Geometry check sheet. Reference: the model listing, model coordinates, mm. A direction names the side the tool comes from. Give positions to 0.01 mm unless a question says otherwise; leave off trailing zeros. Loops run counter-clockwise (first coordinate to the right, second up) from the corner with the lowest first, then second, coordinate; pieces in that order, holes last.
```python
from build123d import *

# Parameters (mm, degrees)
SKETCH1_R           = 10.9
SKETCH1_R_2         = 4
BOSS_EXTRUDE1_DEPTH = 5


with BuildPart() as part:
    # Sketch1 → Boss-Extrude1 (new body)
    with BuildSketch(Plane.XY):
        Circle(SKETCH1_R)
        Circle(SKETCH1_R_2, mode=Mode.SUBTRACT)
    extrude(amount=BOSS_EXTRUDE1_DEPTH)

    # Sketch2 → Cut-Revolve1 (revolve, cut)
    with BuildSketch(Plane(origin=(0, 0, 0), x_dir=(1, 0, 0), z_dir=(0, 1, 0))):
        Polygon((-10.9, -5), (-9.912939245, -5), (-9.732966379, -4.586942685), (-9.293313352, -4.586942685), (-9.243161822, -4.682862035), (-8.878748767, -4.409552244), (-8.742093871, -4.409552244), (-8.742093871, -4.682862035), (-8.362496939, -4.682862035), (-8.302955146, -4.546207139), (-4.812245389, -4.546207139), (-4.748734143, -4.667678158), (-4.635669369, -4.667678158), (-4.635669369, -4.21672133), (-4.317834685, -4.21672133), (-4.317834685, -5), (-6.380746686, -5.704606556), (-10.9, -5.809210272), align=None)
        Polygon((-6.380746686, 0.704606556), (-4.317834685, 0), (-4.317834685, -0.78327867), (-4.635669369, -0.78327867), (-4.635669369, -0.332321842), (-4.748734143, -0.332321842), (-4.812245389, -0.453792861), (-8.302955146, -0.453792861), (-8.362496939, -0.317137965), (-8.742093871, -0.317137965), (-8.742093871, -0.590447756), (-8.878748767, -0.590447756), (-9.243161822, -0.317137965), (-9.293313352, -0.413057315), (-9.732966379, -0.413057315), (-9.912939245, 0), (-10.9, 0), (-10.9, 0.809210272), align=None)
    revolve(axis=Axis((0, 0, 0), (0, 0, 1)), mode=Mode.SUBTRACT)


solid = part.part
```
1) Sectioned sample at A-A on z = 3.95. Enter the section's corners in (x, y), plus the area to 3 significant figures.
2) Depth check by flat-ended pin: P1, Ø2, axis at y = 2.5, z = 1, coming from the -X side. Enter the tip coordinate at first touch or a pass-through.
3) Scan lines: line 1 along Y through (x, z) = (0, 0.7); line 2 along Y through (x, z) = (0, 1.9); line 3 along Y through (x, z) = (0, 4.5). Record each from-to range of solid material in increasing order.
4) Tool access check on faces 3 (the flat face through (-4, -2, 0.783)), 4 (the flat face through (2, -10, 5)). Record the directions out of +Z, -Z, +X, -X, +Y, -Y that give a thin tool (end or side, any length) a straight path to the whole face; none if there is none.
5) Mould release check, pull along Y, two halves, no side actions. Record for faces 1 (the flat face through (2, -10, 0)), 2 (the cylindrical face through (0.936, 4.215, 0.397)): +Y half, -Y half, draft (parallel to the pull), parting line (faces both ways), or undercut.
Determined:
1. outline: circle Ø21.8 at (0, 0); hole circle Ø8 at (0, 0)
1. area: 323 mm2
2. P1: stops at x = -10.8
3. line 1: y = -10.9 to -4.64, -4.32 to -4, 4 to 4.32, 4.64 to 10.9
3. line 2: y = -10.9 to -4, 4 to 10.9
3. line 3: y = -10.9 to -9, -8.74 to -4.64, -4.32 to -4, 4 to 4.32, 4.64 to 8.74, 9 to 10.9
4. face 3: -Z
4. face 4: +Z, +X, -X, +Y, -Y
5. face 1: draft
5. face 2: undercut
